from build123d import *

# Parameters (mm, degrees)
SKETCH1_R            = 16.5
SKETCH1_R_2          = 15
BOSS_EXTRUDE3_DEPTH  = 7
SKETCH2_R            = 27.5
SKETCH2_R_2          = 16.5
BOSS_EXTRUDE4_DEPTH  = 45
SKETCH4_R            = 10
SKETCH4_R_2          = 13
BOSS_EXTRUDE10_DEPTH = 20
BOSS_EXTRUDE11_DEPTH = 7
BOSS_EXTRUDE12_DEPTH = 7
BOSS_EXTRUDE13_DEPTH = 7


with BuildPart() as part:
    # Sketch1 → Boss-Extrude3 (new body)
    with BuildSketch(Plane.XY):
        with BuildLine():
            Line((-322.811275448, 54.020092964), (-308.016991909, 51.544375984))
            ThreePointArc((-308.016991909, 51.544375984), (-297.979605272, 15.041649319), (-263.634141291, -0.882774953))
            Line((-263.634141291, -0.882774953), (-262.985194212, -0.878095462))
            ThreePointArc((-262.985194212, -0.878095462), (-234.213459723, 10.066916736), (-219.209238471, 36.945892575))
            ThreePointArc((-219.209238471, 36.945892575), (-5.54789332, 226.171081865), (222.17000985, 54.119057031))
            ThreePointArc((222.17000985, 54.119057031), (271.744200091, 2.083431527), (308.115870104, 64.070593748))
            Line((308.115870104, 64.070593748), (322.942948353, 66.658271071))
            ThreePointArc((322.942948353, 66.658271071), (72.802770658, 324.018256719), (-281.327086526, 382.296168148))
            ThreePointArc((-281.327086526, 382.296168148), (-317.291599122, 361.87304371), (-330.761322011, 322.769121357))
            Line((-330.761322011, 322.769121357), (-322.811275448, 54.020092964))
        make_face()
        with Locations((-263.634141291, 44.117225047)):
            Circle(SKETCH1_R, mode=Mode.SUBTRACT)
        with Locations((266.5683015, 46.784774614)):
            Circle(SKETCH1_R, mode=Mode.SUBTRACT)
        with Locations((-186.584414745, 266.470160007)):
            Circle(SKETCH1_R_2, mode=Mode.SUBTRACT)
        with Locations((-272.286901184, 324.498892702)):
            Circle(SKETCH1_R_2, mode=Mode.SUBTRACT)
    extrude(amount=BOSS_EXTRUDE3_DEPTH)

    # Sketch2 → Boss-Extrude4 (add)
    with BuildSketch(Plane.XY.offset(7)):
        with Locations((-263.634141291, 44.117225047)):
            Circle(SKETCH2_R)
        with Locations((-263.634141291, 44.117225047)):
            Circle(SKETCH2_R_2, mode=Mode.SUBTRACT)
        with Locations((266.5683015, 46.784774614)):
            Circle(SKETCH2_R)
        with Locations((266.5683015, 46.784774614)):
            Circle(SKETCH2_R_2, mode=Mode.SUBTRACT)
    extrude(amount=-BOSS_EXTRUDE4_DEPTH)

    # Sketch4 → Boss-Extrude10 (add)
    with BuildSketch(Plane(origin=(0, 0, 0), x_dir=(-1, 0, 0), z_dir=(0, 0, -1))):
        with Locations((-73.977350909, 283.959387959)):
            Circle(SKETCH4_R)
        with Locations((77.070617643, 306.793749247)):
            Circle(SKETCH4_R)
        with Locations((0, 304.731170723)):
            Circle(SKETCH4_R_2)
    extrude(amount=BOSS_EXTRUDE10_DEPTH)

    # Sketch6 → Boss-Extrude11 (add)
    with BuildSketch(Plane(origin=(0, 0, 0), x_dir=(-1, 0, 0), z_dir=(0, 0, -1))):
        Polygon((-244.528320181, 186.784774614), (-312.13241104, 86.784774614), (-330.534833245, 103.93991663), (-274.528320181, 186.784774614), align=None)
    extrude(amount=-BOSS_EXTRUDE11_DEPTH)

    # Sketch9 → Boss-Extrude12 (add)
    with BuildSketch(Plane(origin=(0, 0, 0), x_dir=(-1, 0, 0), z_dir=(0, 0, -1))):
        Polygon((326.306060919, 172.160306644), (346.306060919, 172.160306644), (346.306060919, 72.160306644), (323.347893363, 72.160306644), align=None)
    extrude(amount=-BOSS_EXTRUDE12_DEPTH)

    # Sketch10 → Boss-Extrude13 (add)
    with BuildSketch(Plane(origin=(0, 0, 0), x_dir=(-1, 0, 0), z_dir=(0, 0, -1))):
        Polygon((163.634141291, 388.447481806), (163.634141291, 408.447481806), (263.634141291, 408.447481806), (263.634141291, 384.173082441), align=None)
    extrude(amount=-BOSS_EXTRUDE13_DEPTH)


solid = part.part
Design review of the part built by this model. Coordinates are the model's own, in mm. A direction names the side the tool comes from. Coordinates: 2 decimals unless noted, no trailing zeros. Loops run counter-clockwise (first coordinate to the right, second up) from the corner with the lowest first, then second, coordinate; pieces in that order, holes last. Notation, with made-up numbers: M -37,-37 L 0,-37 A21 ccw 0,-31 Z; hole C 82.5,80 d9. An arc over 180 degrees is marked long. Use one line per item in the form item = value.
(1) Consider section C-C (x = 0). Write out the cut boundary in (y, z), and give its area (3 significant figures).
Return value:
outline = M 226.32,0 L 291.73,0 L 291.73,-20 L 317.73,-20 L 317.73,0 L 355.84,0 L 355.84,7 L 226.32,7 Z
area = 1,430 mm2
(2) Consider section D-D (x = 267). Write out the cut boundary in (y, z), and give its area (3 significant figures).
Return value:
outline = M 1.79,0 L 19.29,0 L 19.29,-38 L 30.29,-38 L 30.29,7 L 1.79,7 Z; M 63.28,-38 L 74.28,-38 L 74.28,0 L 186.78,0 L 186.78,7 L 63.28,7 Z
area = 1,900 mm2
(3) Consider section A-A (z = -10). Write out the cut boundary in (x, y).
Return value:
outline = C -263.63,44.12 d55; C -77.07,306.79 d20; C 0,304.73 d26; C 73.98,283.96 d20; C 266.57,46.78 d55; hole C -263.63,44.12 d33; hole C 266.57,46.78 d33
(4) Draft analysis for pull direction X (two halves, no side actions). For faces 4 (the face through (0, 305, -20)), 5 (the face through (-201.57, 267.13, 3.45)), 6 (the face through (321.381, 95.406, 3.451)), state which applies: pulls with the +X half, pulls with the -X half, needs draft (parallel to the pull), parting line crosses it, or undercut.
Return value:
face_4 = needs draft
face_5 = undercut
face_6 = pulls with the +X half
(5) Consider section B-B (x = -184). Write out the cut boundary in (y, z), and give its area (3 significant figures).
Return value:
outline = M 126.39,0 L 251.69,0 L 251.69,7 L 126.39,7 Z; M 281.25,0 L 408.45,0 L 408.45,7 L 281.25,7 Z
area = 1,770 mm2
(6) For line 1 along X through (y, z) = (36, 0.5); line 2 along X through (y, z) = (283.5, -18.5); line 3 along Z through (x, y) = (-304, 133), list the stretches that pass through material, from the lowest coordinate up. Write a range as from..to.
Return value:
line_1 = -307.9..-278, -249.27..-219.37, 222.88..254.08, 279.06..310.26
line_2 = 63.99..83.97
line_3 = 0..7
(7) Clearance check with flat-ended pins moving along their axes: P1, Ø3.5, axis at y = 397.5, z = 2.5, coming from the +X side; P2, Ø5, axis at x = 193.5, z = -0.5, coming from the -Y side; P3, Ø6, axis at y = 167.5, z = -2, coming from the -X side; P4, Ø2, axis at x = 267, z = 4.5, coming from the +Y side. State where each tip first meets the part, or that it passes through.
Return value:
P1 = -163.63
P2 = 117.71
P3 = -346.31
P4 = 186.78
(8) For faces 1 (the face through (302.924, 144.782, 3.451)), 2 (the face through (2.82, 292.04, -9.86)), 3 (the face through (-234.55, 9.78, 3.45)), list the 3-axis set-ups (+Z, -Z, +X, -X, +Y, -Y) from which the entire face can be reached by the end or side of a thin tool; tool diameter is ignored.
Return value:
face_1 = +Z, -Z, +X, +Y
face_2 = -Z
face_3 = +Z, -Z, -Y
